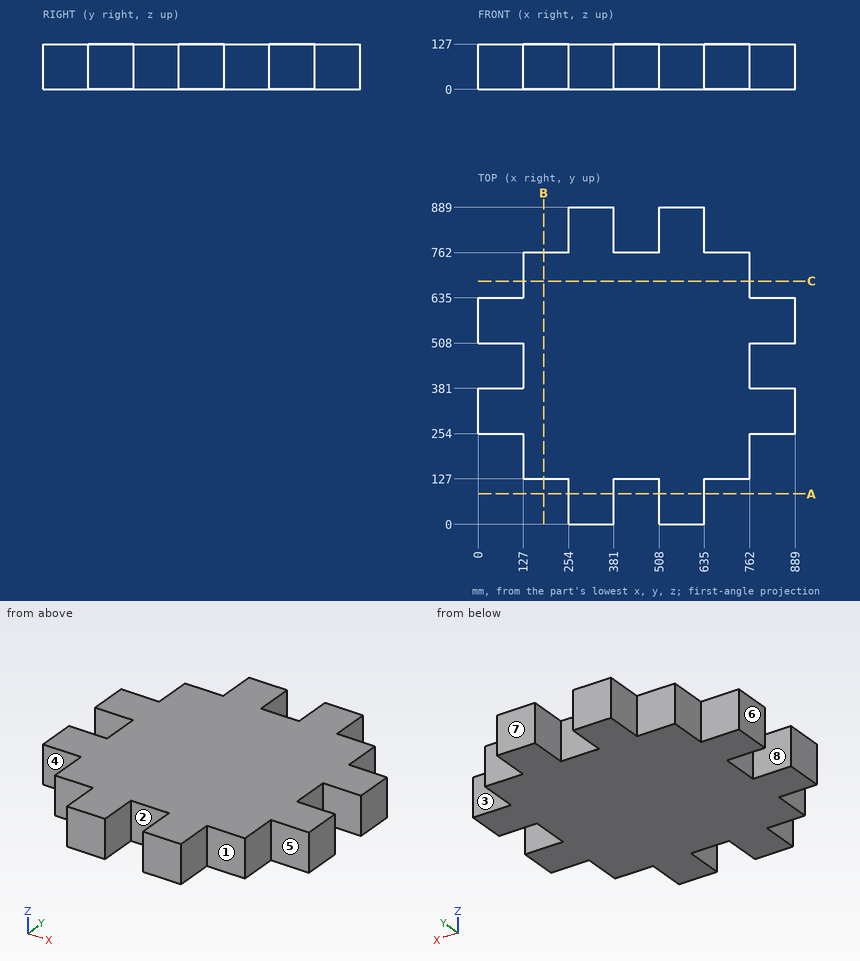
Source: three-view drawing plus pictorial views. Frame: mm from the lowest corner of the part. A direction names the side the tool comes from. Round coordinates to 2 decimals unless told otherwise and drop trailing zeros. Loops run counter-clockwise (first coordinate to the right, second up) from the corner with the lowest first, then second, coordinate; pieces in that order, holes last.
Q1. Ray query, line 1 (X direction, y = 793.5, z = 65.5); line 2 (Y direction, x = 704, z = 51.5). Return the intervals inside material, ascending.
Q2. Section A-A, the plane y = 85. Return loops of the section in (x, z), plus the area to 3 significant figures.
Q3. First-contact query: P1, Ø1.5, axis at x = 119.5, z = 76, coming from the -Y side; P2, Ø10, axis at y = 447.5, z = 113.5, coming from the +X side. Flat tips, straight axial feed; report the tip coordinate or a pass-through.
Q4. Section B-B, the plane x = 184. Return loops of the section in (y, z).
Q5. Mould query, pull axis Y, two halves, no side actions, for the marked faces 5, 6, 7 and 8. Classes: pulls with the +Y half, pulls with the -Y half, needs draft (parallel to the pull), parting line crosses it, or undercut.
Q6. Access query for the marked faces 1, 2, 3 and 4. Directions: +Z, -Z, +X, -X, +Y, -Y. A direction counts if a zero-diameter tool reaches every point of the face in a straight line with its end or side. Return the directions, or none.
Solutions:
1. line 1: x = 254 to 381, 508 to 635
1. line 2: y = 127 to 762
2. outline: (254, 0) - (381, 0) - (381, 127) - (254, 127) - close; (508, 0) - (635, 0) - (635, 127) - (508, 127) - close
2. area: 32,300 mm2
3. P1: stops at y = 254
3. P2: stops at x = 762
4. outline: (127, 0) - (762, 0) - (762, 127) - (127, 127) - close
5. face 5: pulls with the -Y half
5. face 6: needs draft
5. face 7: pulls with the +Y half
5. face 8: undercut
6. face 1: +Z, -Z, +X, -Y
6. face 2: +Z, -Z, -Y
6. face 3: +Z, -Z, +X, +Y
6. face 4: +Z, -Z, -X, -Y
